Could you check a few things on this model? Use its own coordinates, in mm. A direction names the side the tool comes from. Coordinates: 2 decimals unless noted, no trailing zeros. Order: outer loops, then holes, each group sorted by start corner. A loop starts at its lowest first (then second) coordinate and runs counter-clockwise, first axis right, second up. Notation, with made-up numbers: (79.5, 83) -> (87.5, 83) arc R22 ccw to (87.5, 113) -> close; hole circle Ø10 at (83, -26.5). An arc over 180 degrees is marked (long way). Put each result on its own line as item: value. Start each with the question number.
Q1. We'd pull the mould along Y, two halves only. Please class faces 4 (the face through (-53.99, 1.48, 15.04)), 5 (the face through (-1.48, 22.51, -41.11)), 6 (the face through (-54, 0, -31)), 7 (the face through (-1.5, 18.5, -34)): +Y half, -Y half, draft (parallel to the pull), parting line (faces both ways), or undercut.
Q2. Please list where these lines run through material, in increasing order: line 1 along X through (y, z) = (8, -35); line 2 along Z through (x, y) = (-53, 2); line 3 along Y through (x, z) = (-1.7, -40).
Q3. If we section it at A-A (x = -21.5): Please give me the cut outline in (y, z), and give its area (3 significant figures).
Q4. Will these pins go through, and if not, where does the flat tip stop? pin 1 (12 mm diameter, centred on x = -17, z = -22.5, fed in from +Y); pin 2 (4 mm diameter, centred on y = 21.5, z = -6, fed in from -X); pin 3 (2.5 mm diameter, centred on y = 21.5, z = -6, fed in from +X); pin 4 (5 mm diameter, centred on x = -101.5, y = 7.5, fed in from -Z).
Q5. For faces 1 (the face through (-3, 15, -30)), 2 (the face through (-100, 6, 0)), 3 (the face through (-41.92, 1.48, -41.23)), which set-ups out of +Z, -Z, +X, -X, +Y, -Y let a thin tool reach every point of the face, with its end or its side?
Q6. If we section it at C-C (z = -67): Please give me the cut outline in (x, y), and give its area (3 significant figures).
Q7. If we section it at B-B (y = 21.5): Count the separate pieces of the cut face and the enclosed holes in it, and give its area (3 significant figures).
from build123d import *

# Parameters (mm, degrees)
SKETCH1_R            = 4.2
BOSS_EXTRUDE1_DEPTH  = 3
FILLET1_R            = 2
SKETCH2_R            = 1.5
SKETCH2_R_2          = 5
BOSS_EXTRUDE2_DEPTH  = 3
BOSS_EXTRUDE3_DEPTH  = 5
MIRROR3_COPY_1_DEPTH = 5
FILLET2_R            = 4


with BuildPart() as part:
    # Sketch1 → Boss-Extrude1 (new body)
    with BuildSketch(Plane(origin=(0, 0, 0), x_dir=(1, 0, 0), z_dir=(0, 1, 0))):
        with BuildLine():
            Line((-107, 60), (-107, 0))
            Line((-107, 0), (-83.5, 0))
            ThreePointArc((-83.5, 0), (-53.5, -15.042526813), (-23.5, 0))
            Line((-23.5, 0), (0, 0))
            Line((0, 0), (0, 60))
            Line((0, 60), (-23.5, 60))
            ThreePointArc((-23.5, 60), (-53.5, 75.042526813), (-83.5, 60))
            Line((-83.5, 60), (-107, 60))
        make_face()
        Polygon((-97, 45), (-65.5, 30), (-97, 15), align=None, mode=Mode.SUBTRACT)
        Polygon((-83.5, 10), (-53.5, 24.285714286), (-23.5, 10), align=None, mode=Mode.SUBTRACT)
        Polygon((-10, 15), (-41.5, 30), (-10, 45), align=None, mode=Mode.SUBTRACT)
        Polygon((-23.5, 50), (-53.5, 35.714285714), (-83.5, 50), align=None, mode=Mode.SUBTRACT)
        with BuildLine():
            ThreePointArc((-53.5, 62.8), (-57.7, 67), (-53.5, 71.2))
            ThreePointArc((-53.5, 71.2), (-49.3, 67), (-53.5, 62.8))
        make_face(mode=Mode.SUBTRACT)
        with Locations((-53.5, -7)):
            Circle(SKETCH1_R, mode=Mode.SUBTRACT)
    extrude(amount=BOSS_EXTRUDE1_DEPTH)

    # Fillet1
    fillet1_edges = [part.edges().sort_by_distance(p)[0] for p in [
        (-10, 1.5, -15),
        (-10, 1.5, -45),
        (-41.5, 1.5, -30),
        (-83.5, 1.5, -10),
        (-23.5, 1.5, -10),
        (-53.5, 1.5, -24.285714286),
        (-97, 1.5, -45),
        (-97, 1.5, -15),
        (-65.5, 1.5, -30),
        (-23.5, 1.5, -50),
        (-83.5, 1.5, -50),
        (-53.5, 1.5, -35.714285714),
    ]]
    fillet(fillet1_edges, radius=FILLET1_R)

    # Sketch2 → Boss-Extrude2 (add)
    with BuildSketch(Plane.ZY.offset(107)):
        with BuildLine():
            Line((0, 26.5), (-26.077953741, 34.417722444))
            ThreePointArc((-26.077953741, 34.417722444), (-30, 35), (-33.922046259, 34.417722444))
            Line((-33.922046259, 34.417722444), (-60, 26.5))
            Line((-60, 26.5), (-60, 3))
            Line((-60, 3), (0, 3))
            Line((0, 3), (0, 26.5))
        make_face()
        with Locations((-40, 21.5)):
            Circle(SKETCH2_R, mode=Mode.SUBTRACT)
        with Locations((-30, 21.5)):
            Circle(SKETCH2_R_2, mode=Mode.SUBTRACT)
        with Locations((-12, 21.5)):
            Circle(SKETCH2_R, mode=Mode.SUBTRACT)
        with Locations((-6, 21.5)):
            Circle(SKETCH2_R, mode=Mode.SUBTRACT)
        with Locations((-54, 21.5)):
            Circle(SKETCH2_R, mode=Mode.SUBTRACT)
        with Locations((-48, 21.5)):
            Circle(SKETCH2_R, mode=Mode.SUBTRACT)
        with Locations((-20, 21.5)):
            Circle(SKETCH2_R, mode=Mode.SUBTRACT)
    boss_extrude2 = extrude(amount=-BOSS_EXTRUDE2_DEPTH)

    # Mirror1: Boss-Extrude2 across plane
    add(boss_extrude2.mirror(Plane(origin=(-53.5, 0, 0), x_dir=(0, 0, 1), z_dir=(1, 0, 0))))

    # Sketch4 → Boss-Extrude3 (add)
    with BuildSketch(Plane.XY):
        Polygon((-104, 13.5), (-93.75, 3), (-104, 3), align=None)
    boss_extrude3 = extrude(amount=-BOSS_EXTRUDE3_DEPTH)

    # Mirror2: Boss-Extrude3 across plane
    add(boss_extrude3.mirror(Plane(origin=(-53.5, 0, 0), x_dir=(0, 0, 1), z_dir=(1, 0, 0))))

    # Mirror3: Boss-Extrude3 across plane
    add(boss_extrude3.mirror(Plane.XY.offset(-30)))

    # Mirror3 copy 1 sketch → Mirror3 copy 1 (add)
    with BuildSketch(Plane(origin=(-107, 0, -60), x_dir=(-1, 0, 0), z_dir=(0, 0, -1))):
        Polygon((-104, 13.5), (-93.75, 3), (-104, 3), align=None)
    extrude(amount=-MIRROR3_COPY_1_DEPTH)

    # Fillet2
    fillet2_edges = [part.edges().sort_by_distance(p)[0] for p in [
        (-104, 3, -30),
        (-3, 3, -30),
    ]]
    fillet(fillet2_edges, radius=FILLET2_R)


solid = part.part
The answers:
1. face 4: draft
1. face 5: undercut
1. face 6: -Y half
1. face 7: undercut
2. line 1: -107 to -104, -3 to 0
2. line 2: -75.04 to -71.17, -62.83 to -50, -35.99 to -24.01, -10 to 2.83, 11.17 to 15.04
2. line 3: 0 to 20, 23 to 32.57
3. outline: (0, -60) -> (3, -60) -> (3, -39.52) -> (0, -39.52) -> close; (0, -20.48) -> (3, -20.48) -> (3, 0) -> (0, 0) -> close
3. area: 123 mm^2
4. pin 1: y = 3
4. pin 2: x = -107
4. pin 3: through
4. pin 4: z = -60
5. face 1: +Y
5. face 2: +Z, -X, +Y, -Y
5. face 3: +Y, -Y
6. outline: (-76.68, 0) -> (-57.7, 0) -> (-57.7, 3) -> (-76.68, 3) -> close; (-49.3, 0) -> (-30.32, 0) -> (-30.32, 3) -> (-49.3, 3) -> close
6. area: 114 mm^2
7. separate pieces: 16
7. enclosed holes: 0
7. area: 192 mm^2
